For this review, take the finished solid that the model builds, in its own axes (mm). Coordinates: 2 decimals unless noted, no trailing zeros. Put each result on its own line as item: value. Start each with the question number.
Item 1: To check wall thickness, follow L1, parallel to Y at x = 8, z = 280; L2, parallel to Y at x = 7, z = 357.5; L3, parallel to X at y = -4.75, z = 156. State the ranges of each line that lie inside material, in increasing order.
Item 2: Insertion check: P1, Ø6, axis at x = 1, z = 172, coming from the -Y side; P2, Ø1.5, axis at x = 0, z = 263.5, coming from the -Y side; P3, Ø1.5, axis at x = -0.5, z = 380.5, coming from the +Y side. Each pin has a flat end and moves straight along its axis. Give the tip position at first contact, or say it passes through.
Item 3: Consider section A-A on z = 94. Give the number of separate pieces and of enclosed holes in the cut face, and give its area (3 significant figures).
Autodesk Inventor part; units mm, degrees
ref_plane "Start Plane" through (0, 0, 0) normal (0, 0, 1) x (1, 0, 0)
ref_plane "End Plane" through (0, 0, 550) normal (0, 0, 1) x (1, 0, 0)
ref_plane "YZ Plane" through (0, 0, 0) normal (1, 0, 0) x (0, 1, 0)
ref_plane "Start Plane" through (0, 0, 0) normal (0, 0, 1) x (1, 0, 0)
ref_plane "End Plane" through (0, 0, 550) normal (0, 0, 1) x (1, 0, 0)
sketch "Sketch1" plane through (0, 0, 0) normal (0, 0, 1) x (1, 0, 0)
  line L0 (10, -4.5951) -> (10, -8.2)
  line L1 (-10, -8.2) -> (-10, -4.5951)
  line L2 (-10, 10) -> (10, -10) construction
  line L3 (10, 10) -> (-10, -10) construction
  circle A0 centre (0, 0) radius 2.1
  line L4 (-2.84, -3.9007) -> (2.84, -3.9007)
  line L5 (3.9007, -2.84) -> (3.9007, 2.84)
  line L6 (2.84, 3.9007) -> (-2.84, 3.9007)
  line L7 (-3.9007, 2.84) -> (-3.9007, -2.84)
  line L8 (-3.9007, -3.9007) -> (3.9007, 3.9007) construction
  line L9 (3.9007, -3.9007) -> (-3.9007, 3.9007) construction
  line L10 (-3.9007, -2.84) -> (-2.84, -3.9007) construction
  line L11 (-2.84, -3.9007) -> (-5.4993, -6.56)
  line L12 (-5.4993, -6.56) -> (-5.4993, -8.2)
  line L13 (-5.4993, -8.2) -> (-2.7951, -8.2)
  line L14 (-2.7951, -8.2) -> (-4.5951, -10)
  line L15 (0, 0) -> (0, -3.9007) construction
  line L16 (3.9007, -2.84) -> (2.84, -3.9007) construction
  line L17 (2.84, -3.9007) -> (5.4993, -6.56)
  line L18 (5.4993, -6.56) -> (5.4993, -8.2)
  line L19 (5.4993, -8.2) -> (2.7951, -8.2)
  line L20 (2.7951, -8.2) -> (4.5951, -10)
  line L21 (-2.84, -3.9007) -> (-3.9007, -2.84) construction
  line L22 (-3.9007, -2.84) -> (-6.56, -5.4993)
  line L23 (-6.56, -5.4993) -> (-8.2, -5.4993)
  line L24 (-8.2, -5.4993) -> (-8.2, -2.7951)
  line L25 (-8.2, -2.7951) -> (-10, -4.5951)
  line L26 (3.9007, -2.84) -> (6.56, -5.4993)
  line L27 (6.56, -5.4993) -> (8.2, -5.4993)
  line L28 (8.2, -5.4993) -> (8.2, -2.7951)
  line L29 (8.2, -2.7951) -> (10, -4.5951)
  arc A1 (-10, -8.2) -> (-8.2, -10) centre (-8.2, -8.2) ccw
  arc A2 (8.2, -10) -> (10, -8.2) centre (8.2, -8.2) ccw
  line L30 (-8.2, -6.56) -> (-7.7111, -6.56)
  line L31 (-6.6505, -8.2) -> (-8.2, -8.2)
  line L32 (-8.2, -8.2) -> (-8.2, -6.56)
  line L33 (-6.6505, -7.6207) -> (-7.7111, -6.56)
  line L34 (-6.6505, -7.6207) -> (-6.6505, -8.2)
  line L35 (8.2, -6.56) -> (7.7111, -6.56)
  line L36 (6.6505, -8.2) -> (8.2, -8.2)
  line L37 (8.2, -8.2) -> (8.2, -6.56)
  line L38 (6.6505, -7.6207) -> (7.7111, -6.56)
  line L39 (6.6505, -7.6207) -> (6.6505, -8.2)
  line L40 (8.2, -10) -> (4.5951, -10)
  line L41 (-4.5951, -10) -> (-8.2, -10)
  line L42 (-3.9007, 0) -> (3.9007, 0) construction
  line L43 (10, 4.5951) -> (10, 8.2)
  line L44 (-10, 8.2) -> (-10, 4.5951)
  line L45 (-2.84, 3.9007) -> (2.84, 3.9007)
  line L46 (-3.9007, 2.84) -> (-2.84, 3.9007) construction
  line L47 (-2.84, 3.9007) -> (-5.4993, 6.56)
  line L48 (-5.4993, 6.56) -> (-5.4993, 8.2)
  line L49 (-5.4993, 8.2) -> (-2.7951, 8.2)
  line L50 (-2.7951, 8.2) -> (-4.5951, 10)
  line L51 (2.84, 3.9007) -> (5.4993, 6.56)
  line L52 (5.4993, 6.56) -> (5.4993, 8.2)
  line L53 (5.4993, 8.2) -> (2.7951, 8.2)
  line L54 (2.7951, 8.2) -> (4.5951, 10)
  line L55 (3.9007, 2.84) -> (2.84, 3.9007) construction
  line L56 (-8.2, 2.7951) -> (-10, 4.5951)
  line L57 (-2.84, 3.9007) -> (-3.9007, 2.84) construction
  line L58 (-3.9007, 2.84) -> (-6.56, 5.4993)
  line L59 (-6.56, 5.4993) -> (-8.2, 5.4993)
  line L60 (-8.2, 5.4993) -> (-8.2, 2.7951)
  line L61 (3.9007, 2.84) -> (6.56, 5.4993)
  line L62 (6.56, 5.4993) -> (8.2, 5.4993)
  line L63 (8.2, 5.4993) -> (8.2, 2.7951)
  line L64 (8.2, 2.7951) -> (10, 4.5951)
  arc A3 (-8.2, 10) -> (-10, 8.2) centre (-8.2, 8.2) ccw
  arc A4 (10, 8.2) -> (8.2, 10) centre (8.2, 8.2) ccw
  line L65 (-8.2, 6.56) -> (-7.7111, 6.56)
  line L66 (-6.6505, 8.2) -> (-8.2, 8.2)
  line L67 (-8.2, 8.2) -> (-8.2, 6.56)
  line L68 (-6.6505, 7.6207) -> (-7.7111, 6.56)
  line L69 (-6.6505, 7.6207) -> (-6.6505, 8.2)
  line L70 (8.2, 6.56) -> (7.7111, 6.56)
  line L71 (6.6505, 7.6207) -> (7.7111, 6.56)
  line L72 (8.2, 8.2) -> (8.2, 6.56)
  line L73 (6.6505, 7.6207) -> (6.6505, 8.2)
  line L74 (6.6505, 8.2) -> (8.2, 8.2)
  line L75 (8.2, 10) -> (4.5951, 10)
  line L76 (-4.5951, 10) -> (-8.2, 10)
  line L77 (-8.2, 10) -> (-4.5951, 10)
  line L78 (4.5951, 10) -> (8.2, 10)
  point P0 (8.2, -8.2)
  point P1 (0, 3.9007)
  point P2 (8.2, 8.2)
  dimension "Width" = 20
  dimension "Height" = 20
  dimension "d2" = 4.2
  dimension "d3" = 1.5
  dimension "d4" = 1.64
  dimension "d6" = 5.68
  dimension "d7" = 1.8
  dimension "d9" = 1.5
extrude "Body" add sketch "Sketch1" along normal up to surface (550 mm away) from surface at 0
sketch "Sketch4" plane through (0, 0, 0) normal (0, 0, 1) x (1, 0, 0)
  line L0 (0, 0) -> (10, 0)
ref_plane "Work Plane4" through (0, 0, 0) normal (0, -1, 0) x (1, 0, 0)
sketch "Sketch5" plane through (0, 0, 0) normal (0, -1, 0) x (1, 0, 0)
  line L0 (-2, 0) -> (12, 0) construction
  line L1 (-2, 550) -> (12, 550) construction
  dimension "d17" = 550
equation "\"G_OFFSET_START\" = 0"
equation "\"G_OFFSET_END\" = 0"
equation "\"G_L\" = d17"
properties part number "V-slot 20 mm x 20 mm" material "Aluminum 6061"
Return value:
1. L1: -10 to -8.2, -6.56 to -5.5, 5.5 to 6.56, 8.2 to 10
1. L2: -10 to -8.2, -7.27 to -5.5, 5.5 to 7.27, 8.2 to 10
1. L3: -10 to -8.2, -5.81 to -3.69, 3.69 to 5.81, 8.2 to 10
2. P1: y = -9.4
2. P2: y = -3.9
2. P3: y = 3.9
3. separate pieces: 1
3. enclosed holes: 5
3. area: 161 mm^2
